Read the model definition and answer for the solid it produces. Units are mm, in the model's axes. Round coordinates to 2 decimals unless told otherwise and drop trailing zeros. Write each loop counter-clockwise with the first axis right and the second up, starting at its lowest first coordinate (ties: lowest second). Pieces come first, ordered by that corner, then holes.
from build123d import *

# Parameters (mm, degrees)
SKETCH1_W           = 70
SKETCH1_H           = 120
SKETCH1_R           = 2.5
SKETCH1_R_2         = 2.85
BOSS_EXTRUDE1_DEPTH = 8
SKETCH2_R           = 2.5
CUT_EXTRUDE1_DEPTH  = 93.54188241
SKETCH4_W           = 106.143175547
SKETCH4_H           = 17.825571466
SKETCH4_W_2         = 120.889784669
SKETCH4_H_2         = 15.71891302
CUT_EXTRUDE2_DEPTH  = 93.54188241
SKETCH5_R           = 2.5
CUT_EXTRUDE3_DEPTH  = 87.394444266
SKETCH6_R           = 4.25
CUT_EXTRUDE4_DEPTH  = 6
SKETCH7_R           = 4.25
CUT_EXTRUDE5_DEPTH  = 6


with BuildPart() as part:
    # Sketch1 → Boss-Extrude1 (new body)
    with BuildSketch(Plane.XY):
        with Locations((-35, 0)):
            Rectangle(SKETCH1_W, SKETCH1_H)
        with Locations((-61.5, 37.5)):
            Circle(SKETCH1_R, mode=Mode.SUBTRACT)
        with Locations((-28.5, 37.5)):
            Circle(SKETCH1_R, mode=Mode.SUBTRACT)
        with Locations((-61.5, 11.5)):
            Circle(SKETCH1_R, mode=Mode.SUBTRACT)
        with Locations((-28.5, 11.5)):
            Circle(SKETCH1_R, mode=Mode.SUBTRACT)
        with Locations((-61.5, -11.5)):
            Circle(SKETCH1_R, mode=Mode.SUBTRACT)
        with Locations((-28.5, -11.5)):
            Circle(SKETCH1_R, mode=Mode.SUBTRACT)
        with Locations((-28.5, -37.5)):
            Circle(SKETCH1_R, mode=Mode.SUBTRACT)
        with Locations((-61.5, -37.5)):
            Circle(SKETCH1_R, mode=Mode.SUBTRACT)
        with Locations((-15, 45.1)):
            Circle(SKETCH1_R_2, mode=Mode.SUBTRACT)
        with Locations((-15, 13)):
            Circle(SKETCH1_R_2, mode=Mode.SUBTRACT)
        with Locations((-15, -13)):
            Circle(SKETCH1_R_2, mode=Mode.SUBTRACT)
        with Locations((-15, -45.1)):
            Circle(SKETCH1_R_2, mode=Mode.SUBTRACT)
    extrude(amount=BOSS_EXTRUDE1_DEPTH)

    # Sketch2 → Cut-Extrude1 (cut, through all)
    with BuildSketch(Plane.XY.offset(8)):
        with Locations((-45, 0)):
            Circle(SKETCH2_R)
    extrude(amount=-CUT_EXTRUDE1_DEPTH, mode=Mode.SUBTRACT)

    # Sketch4 → Cut-Extrude2 (cut, through all)
    with BuildSketch(Plane(origin=(0, 0, 0), x_dir=(-1, 0, 0), z_dir=(0, 0, -1))):
        with Locations((33.542634591, 58.912785733)):
            Rectangle(SKETCH4_W, SKETCH4_H)
        with Locations((34.920065114, -57.85945651)):
            Rectangle(SKETCH4_W_2, SKETCH4_H_2)
    extrude(amount=-CUT_EXTRUDE2_DEPTH, mode=Mode.SUBTRACT)

    # Sketch5 → Cut-Extrude3 (cut, through all)
    with BuildSketch(Plane(origin=(0, 0, 0), x_dir=(-1, 0, 0), z_dir=(0, 0, -1))):
        with Locations((59, 0)):
            Circle(SKETCH5_R)
        with Locations((15, 0)):
            Circle(SKETCH5_R)
    extrude(amount=-CUT_EXTRUDE3_DEPTH, mode=Mode.SUBTRACT)

    # Sketch6 → Cut-Extrude4 (cut)
    with BuildSketch(Plane(origin=(0, 0, 0), x_dir=(-1, 0, 0), z_dir=(0, 0, -1))):
        with Locations((28.5, 37.5)):
            Circle(SKETCH6_R)
        with Locations((61.5, 37.5)):
            Circle(SKETCH6_R)
        with Locations((28.5, 11.5)):
            Circle(SKETCH6_R)
        with Locations((61.5, 11.5)):
            Circle(SKETCH6_R)
        with Locations((28.5, -11.5)):
            Circle(SKETCH6_R)
        with Locations((61.5, -11.5)):
            Circle(SKETCH6_R)
        with Locations((61.5, -37.5)):
            Circle(SKETCH6_R)
        with Locations((28.5, -37.5)):
            Circle(SKETCH6_R)
    extrude(amount=-CUT_EXTRUDE4_DEPTH, mode=Mode.SUBTRACT)

    # Sketch7 → Cut-Extrude5 (cut)
    with BuildSketch(Plane(origin=(0, 0, 0), x_dir=(-1, 0, 0), z_dir=(0, 0, -1))):
        with Locations((15, 0)):
            Circle(SKETCH7_R)
        with Locations((59, 0)):
            Circle(SKETCH7_R)
    extrude(amount=-CUT_EXTRUDE5_DEPTH, mode=Mode.SUBTRACT)


solid = part.part
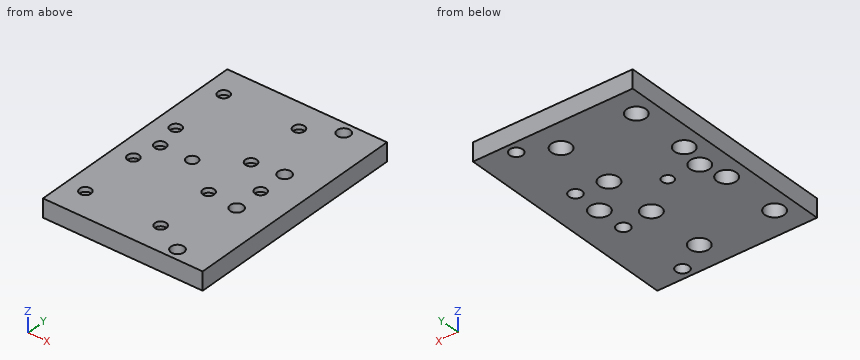
Q1. Section A-A (x = -15) is taken. Determine the outline of the cut face in (y, z), then the cut area to 3 significant figures.
Verdict:
outline: (-50, 0) - (-47.95, 0) - (-47.95, 8) - (-50, 8) - close; (-42.25, 0) - (-15.85, 0) - (-15.85, 8) - (-42.25, 8) - close; (-10.15, 0) - (-4.25, 0) - (-4.25, 6) - (-2.5, 6) - (-2.5, 8) - (-10.15, 8) - close; (2.5, 6) - (4.25, 6) - (4.25, 0) - (10.15, 0) - (10.15, 8) - (2.5, 8) - close; (15.85, 0) - (42.25, 0) - (42.25, 8) - (15.85, 8) - close; (47.95, 0) - (50, 0) - (50, 8) - (47.95, 8) - close
area: 557 mm2
Q2. Straight lines are drawn through the part: probe 1 along Y at (x, z) = (-28.5, 1.85); probe 2 along Y at (x, z) = (-28.5, 7); probe 3 along Y at (x, z) = (-15, 5.5). For each, find the intervals that lie inside material, in ascending order.
Verdict:
probe 1: y = -50 to -41.75, -33.25 to -15.75, -7.25 to 7.25, 15.75 to 33.25, 41.75 to 50
probe 2: y = -50 to -40, -35 to -14, -9 to 9, 14 to 35, 40 to 50
probe 3: y = -50 to -47.95, -42.25 to -15.85, -10.15 to -4.25, 4.25 to 10.15, 15.85 to 42.25, 47.95 to 50
Q3. Section D-D (y = 13) is taken. Determine the outline of the cut face in (x, z).
Verdict:
outline: (-70, 0) - (-65.48, 0) - (-65.48, 6) - (-63.5, 6) - (-63.5, 8) - (-70, 8) - close; (-59.5, 6) - (-57.52, 6) - (-57.52, 0) - (-32.48, 0) - (-32.48, 6) - (-30.5, 6) - (-30.5, 8) - (-59.5, 8) - close; (-26.5, 6) - (-24.52, 6) - (-24.52, 0) - (-17.85, 0) - (-17.85, 8) - (-26.5, 8) - close; (-12.15, 0) - (0, 0) - (0, 8) - (-12.15, 8) - close
Q4. Section B-B (x = -45) is taken. Determine the outline of the cut face in (y, z), then the cut area to 3 significant figures.
Verdict:
outline: (-50, 0) - (-2.5, 0) - (-2.5, 8) - (-50, 8) - close; (2.5, 0) - (50, 0) - (50, 8) - (2.5, 8) - close
area: 760 mm2
Q5. Section C-C (z = 4.5) is taken. State how many separate pieces and enclosed holes the cut face has, then the cut area to 3 significant figures.
Verdict:
separate pieces: 1
enclosed holes: 15
area: 6,310 mm2
Q6. A flat-ended cylindrical pin translates along its axis: pin 1 Ø4 at (x, y) = (-30.5, -37) entering from -Z. Find the tip coordinate at first contact, or state that the pin passes through.
Verdict:
pin 1: stops at z = 6
